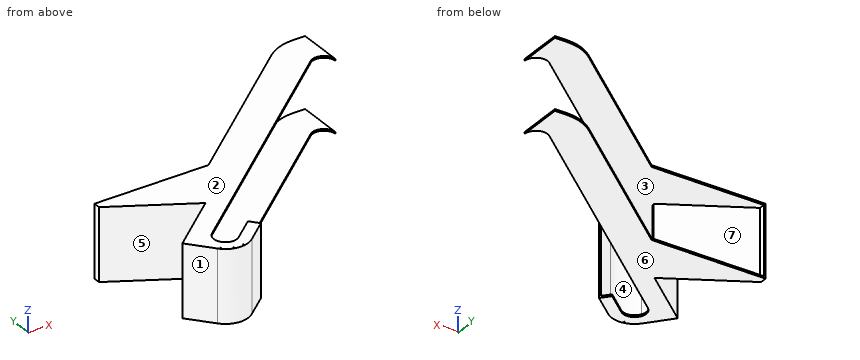
from build123d import *

# Parameters (mm, degrees)
EXTRUDE_1_DEPTH        = 4
PATTERN_LINEAR_1_COUNT = 2
PATTERN_LINEAR_1_PITCH = 310.4
SKETCH_7_W             = 395.874868567
SKETCH_7_H             = 318.4
EXTRUDE_2_DEPTH        = 8
SKETCH_8_W             = 318.4
SKETCH_8_H             = 30
EXTRUDE_3_DEPTH        = 8
SKETCH_9_W             = 298.07386306
SKETCH_9_H             = 318.4
EXTRUDE_4_DEPTH        = 4
EXTRUDE_5_DEPTH        = 318.4


with BuildPart() as part:
    # Sketch 4 → Extrude 1 (new, symmetric)
    with BuildSketch(Plane.XY):
        with BuildLine():
            Line((420.987802859, 562.886051953), (471.987802859, 562.886051953))
            Line((471.987802859, 562.886051953), (471.987802859, 361.886051953))
            ThreePointArc((471.987802859, 361.886051953), (442.540044204, 408.108350608), (388.203454114, 400.952488665))
            Line((388.203454114, 400.952488665), (-607.607677768, -434.726989137))
            ThreePointArc((-607.607677768, -434.726989137), (-613.889765736, -506.577774594), (-542.038980279, -512.859862561))
            Line((-542.038980279, -512.859862561), (-450.117952721, -435.720218456))
            Line((-450.117952721, -435.720218456), (-423.119077284, -467.892578102))
            Line((-423.119077284, -467.892578102), (-515.018746035, -545.014298008))
            ThreePointArc((-515.018746035, -545.014298008), (-582.867486655, -566.333113479), (-645.94139002, -533.475447539))
            Line((-645.94139002, -533.475447539), (-730.152226268, -433.128256555))
            Line((-730.152226268, -433.128256555), (-659.034107171, -373.446304098))
            Line((-659.034107171, -373.446304098), (-501.825094761, -241.51732561))
            Line((-501.825094761, -241.51732561), (-846.623641588, -47.015722354))
            Line((-846.623641588, -47.015722354), (-846.623641588, -17.015722354))
            Line((-846.623641588, -17.015722354), (-343.198253767, -17.015722354))
            Line((-343.198253767, -17.015722354), (291.778898983, 515.853773113))
            ThreePointArc((291.778898983, 515.853773113), (352.236482701, 550.762350034), (420.987802859, 562.886051953))
        make_face()
    extrude(amount=EXTRUDE_1_DEPTH, both=True)


with BuildPart() as pattern_linear_1_1:
    # Pattern Linear 1: pattern copy
    add(part.part.moved(Location(Vector(0, 0, 1) * (1 * PATTERN_LINEAR_1_PITCH))))


with BuildPart() as part_1:
    add(part.part)

    add(pattern_linear_1_1.part)  # Extrude 2 merges Pattern Linear 1_1
    # Sketch 7 → Extrude 2 (add)
    with BuildSketch(Plane(origin=(-224.491205057, -397.961970406, 0), x_dir=(0.870978620276557, -0.4913209165312884, 0), z_dir=(-0.4913209165312884, -0.870978620276557, 0))):
        with Locations((-516.353849163, 155.2)):
            Rectangle(SKETCH_7_W, SKETCH_7_H)
    extrude(amount=-EXTRUDE_2_DEPTH)

    # Sketch 8 → Extrude 3 (add)
    with BuildSketch(Plane.ZY.offset(846.623641588)):
        with Locations((155.2, -32.015722354)):
            Rectangle(SKETCH_8_W, SKETCH_8_H)
    extrude(amount=-EXTRUDE_3_DEPTH)

    # Sketch 9 → Extrude 4 (add, symmetric)
    with BuildSketch(Plane(origin=(-88.443218659, 105.390576195, 0), x_dir=(0.7660085629862927, 0.6428303675400493, 0), z_dir=(-0.6428303675400493, 0.7660085629862927, 0))):
        with Locations((-688.693922428, -155.2)):
            Rectangle(SKETCH_9_W, SKETCH_9_H)
    extrude(amount=EXTRUDE_4_DEPTH, both=True)

    # Sketch 10 → Extrude 5 (add)
    with BuildSketch(Plane.XY.offset(314.4)):
        with BuildLine():
            Line((-732.723547738, -430.064222303), (-645.94139002, -533.475447539))
            ThreePointArc((-645.94139002, -533.475447539), (-582.872198439, -566.386574546), (-515.018746035, -545.014298008))
            Line((-515.018746035, -545.014298008), (-423.119077284, -467.892578102))
            Line((-423.119077284, -467.892578102), (-417.802582401, -473.874750967))
            Line((-417.802582401, -473.874750967), (-509.876103095, -551.142366512))
            ThreePointArc((-509.876103095, -551.142366512), (-583.574554826, -574.355683374), (-652.076622248, -538.609541958))
            Line((-652.076622248, -538.609541958), (-738.851610287, -435.206860245))
            Line((-738.851610287, -435.206860245), (-732.723547738, -430.064222303))
        make_face()
    extrude(amount=-EXTRUDE_5_DEPTH)


solid = part_1.part
Read the model definition and answer for the solid it produces. Units are mm, in the model's axes. Face numbers are marked on the shaded views. A direction names the side the tool comes from. Give positions to 0.01 mm unless a question says otherwise; leave off trailing zeros. Loops run counter-clockwise (first coordinate to the right, second up) from the corner with the lowest first, then second, coordinate; pieces in that order, holes last. Notation, with made-up numbers: (-36, -39.5) - (-14, -39.5) arc R17 ccw to (-14, -13.5) - close; hole circle Ø7 at (-23, 32.5). An arc over 180 degrees is marked (long way). Answer as CSV lines item,"result". Start each with the question number.
1) Which of the six approach directions +Z, -Z, +X, -X, +Y, -Y give full straight-line access (tool end or side, diameter ignored) to the marked faces 4, 5, 6 and 7?
2) Determine the mould class of the marked faces 1, 2 and 3 for opening direction Z: released by +Z, released by -Z, zero draft, split by the parting line, or undercut.
3) Find section C-C (y = 100.5). Write down the section's boundary in (x, z), then the cut area to 3 significant figures.
4) Find section B-B (x = 321.5). Write down the section's boundary in (y, z).
5) Find section D-D (y = -268.5). Write down the section's boundary in (x, z).
6) Straight lines are drawn through the part: L1, parallel to Z at x = -479, y = -159; L2, parallel to Y at x = -530, z = 258; L3, parallel to Y at x = -603, z = 32. For each, find the intervals that lie inside material, in ascending order. Write a range as from..to.
7) Find section A-A (z = 292). Write down the section's boundary in (x, y).
8) Each of these flat-tipped pins is pushed along its axis until it touches: pin 1 Ø10 at (x, z) = (-558, 190.5) entering from -Y; pin 2 Ø7.5 at (y, z) = (-29, 136.5) entering from +X; pin 3 Ø2 at (y, z) = (-351.5, 94) entering from +X. Where does it stop, or does it pass through?
Findings below:
1,face 4,"none"
1,face 5,"+Z, -Z, -X"
1,face 6,"-Z, +X, -X, +Y, -Y"
1,face 7,"+X, +Y"
2,face 1,"zero draft"
2,face 2,"released by +Z"
2,face 3,"undercut"
3,outline,"(-203.16, -4) - (30.18, -4) - (30.18, 4) - (-203.16, 4) - close; (-203.16, 306.4) - (30.18, 306.4) - (30.18, 314.4) - (-203.16, 314.4) - close"
3,area,"3,730 mm^2"
4,outline,"(344.98, -4) - (536.54, -4) - (536.54, 4) - (344.98, 4) - close; (344.98, 306.4) - (536.54, 306.4) - (536.54, 314.4) - (344.98, 314.4) - close"
5,outline,"(-540.2, -4) - (-409.53, -4) - (-409.53, 4) - (-527.76, 4) - (-527.76, 306.4) - (-409.53, 306.4) - (-409.53, 314.4) - (-540.2, 314.4) - close"
6,L1,"-4..4, 306.4..314.4"
6,L2,"-564.29..-555.27, -270.38..-259.94, -225.62..-216.44"
6,L3,"-570.7..-562.33, -331.64..-321.2, -184.44..-175.26"
7,outline,"(-846.62, -47.02) - (-505.55, -239.42) - (-738.85, -435.21) - (-652.08, -538.61) arc R100.87 ccw to (-509.88, -551.14) - (-417.8, -473.87) - (-423.12, -467.89) - (-515.02, -545.01) arc R92.87 cw to (-645.94, -533.48) - (-727.58, -436.19) - (-499.25, -244.58) - (-501.83, -241.52) - (-497.89, -234.55) - (-838.62, -42.34) - (-838.62, -17.02) - (-846.62, -17.02) - close"
8,pin 1,"y = -574.06"
8,pin 2,"x = -838.62"
8,pin 3,"x = -625.47"
